Verification items for the finished model (mm, model axes). A direction names the side the tool comes from. Coordinates: 2 decimals unless noted, no trailing zeros. Write each loop counter-clockwise with the first axis right and the second up, starting at its lowest first coordinate (ties: lowest second). Pieces come first, ordered by that corner, then holes. Notation, with made-up numbers: (2.5, 14.25) -> (52.5, 14.25) arc R22 cw to (52.5, 44.25) -> close; hole circle Ø3 at (19, -6). An arc over 180 degrees is marked (long way). Answer in a Markdown table with one row per item.
```python
from build123d import *

# Parameters (mm, degrees)
BASE_DEPTH                           = 8.2
SIDES_DEPTH                          = 21
F_3_2_3_2_MOUNTING_HOLES_D           = 3.2
F_3_2_3_2_MOUNTING_HOLES_ON_FACE_2_D = 3.2
F_3_2_3_2_MOUNTING_HOLES_ON_FACE_3_D = 3.2
INSIDEFILLET_R                       = 3
OUTSIDEFILLET_R                      = 4
NUTSLOT_START                        = -4
NUTSLOT_DEPTH                        = 3


with BuildPart() as part:
    # Sketch4 → Base (new body)
    with BuildSketch(Plane.XY):
        Polygon((0, 20), (0, 0), (20, 0), (20, 6), (6, 20), align=None)
    extrude(amount=BASE_DEPTH)

    # Sketch4_4 → Sides (add)
    with BuildSketch(Plane.XY):
        Polygon((0, 0), (20, 0), (20, 4), (4, 4), (4, 20), (0, 20), align=None)
    extrude(amount=SIDES_DEPTH)

    # 3.2 _3.2_ Mounting Holes (through all)
    with Locations(Plane(origin=(14, 0, 15), x_dir=(0, 0, -1), z_dir=(0, -1, 0))):
        with Locations((0, 0)):
            Hole(F_3_2_3_2_MOUNTING_HOLES_D / 2)

    # 3.2 _3.2_ Mounting Holes on face 2 (through all)
    with Locations(Plane(origin=(0, 14, 15), x_dir=(0, 0, -1), z_dir=(-1, 0, 0))):
        with Locations((0, 0)):
            Hole(F_3_2_3_2_MOUNTING_HOLES_ON_FACE_2_D / 2)

    # 3.2 _3.2_ Mounting Holes on face 3 (through all)
    with Locations(Plane(origin=(9, 9, 0), x_dir=(-1, 0, 0), z_dir=(0, 0, -1))):
        with Locations((0, 0)):
            Hole(F_3_2_3_2_MOUNTING_HOLES_ON_FACE_3_D / 2)

    # InsideFillet
    insidefillet_edges = [part.edges().sort_by_distance(p)[0] for p in [
        (12, 4, 8.2),
        (4, 4, 14.6),
        (4, 12, 8.2),
    ]]
    fillet(insidefillet_edges, radius=INSIDEFILLET_R)

    # OutsideFillet
    outsidefillet_edges = [part.edges().sort_by_distance(p)[0] for p in [
        (6, 20, 4.185786438),
        (20, 6, 4.185786438),
        (20, 2, 21),
        (2, 20, 21),
    ]]
    fillet(outsidefillet_edges, radius=OUTSIDEFILLET_R)

    # Sketch7 → NutSlot (cut)
    with BuildSketch(Plane(origin=(0, 0, 0), x_dir=(-1, 0, 0), z_dir=(0, 0, -1)).offset(NUTSLOT_START)):
        Polygon((-8.228417185, 17.771582815), (-5.641242789, 8.116116524), (-8.116116524, 5.641242789), (-17.771582815, 8.228417185), align=None)
    extrude(amount=-NUTSLOT_DEPTH, mode=Mode.SUBTRACT)


solid = part.part
```
1. Tool access check on faces 4 (the flat face through (10.3, 10.4, 7)), 5 (the flat face through (13, 13, 3)), 6 (the flat face through (4, 13, 17)). Record the directions out of +Z, -Z, +X, -X, +Y, -Y that give a thin tool (end or side, any length) a straight path to the whole face; none if there is none.
Geometry says:
| item | result |
|---|---|
| face 4 | none |
| face 5 | +Z, -Z, +X, +Y |
| face 6 | +Z, +X, +Y |
2. Section check D-D, the plane y = 14. Record the boundary of the cut face in (x, z), plus the area to 3 significant figures.
Geometry says:
| item | result |
|---|---|
| outline | (0, 0) -> (12, 0) -> (12, 4) -> (7.22, 4) -> (7.22, 7) -> (12, 7) -> (12, 8.2) -> (7, 8.2) arc R3 cw to (4, 11.2) -> (4, 13.4) -> (0, 13.4) -> close; (0, 16.6) -> (4, 16.6) -> (4, 21) -> (0, 21) -> close |
| area | 124 mm^2 |
3. Depth check by flat-ended pin: P1, Ø8, axis at x = 12, z = 8, coming from the +Y side; P2, Ø9.5, axis at x = 15, y = 12, coming from the +Z side; P3, Ø5, axis at x = 11.5, z = 14.5, coming from the +Y side. Enter the tip coordinate at first touch or a pass-through.
Geometry says:
| item | result |
|---|---|
| P1 | y = 18 |
| P2 | z = 8.2 |
| P3 | y = 4 |
4. Thickness scan on line 1 (Y direction, x = 9, z = 7.7); line 2 (Z direction, x = 10.25, y = 11); line 3 (X direction, y = 2.4, z = 15). Record the ranges inside material, lowest first. Write a range as from..to.
Geometry says:
| item | result |
|---|---|
| line 1 | 0..7.4, 10.6..17 |
| line 2 | 0..4, 7..8.2 |
| line 3 | 0..12.4, 15.6..20 |
5. Section check B-B, the plane y = 9. Record the boundary of the cut face in (x, z), plus the area to 3 significant figures.
Geometry says:
| item | result |
|---|---|
| outline | (0, 0) -> (7.4, 0) -> (7.4, 4) -> (5.88, 4) -> (5.88, 7) -> (7.4, 7) -> (7.4, 8.2) -> (7, 8.2) arc R3 cw to (4, 11.2) -> (4, 21) -> (0, 21) -> close; (10.6, 0) -> (17, 0) -> (17, 4) -> (10.6, 4) -> close; (10.6, 7) -> (17, 7) -> (17, 8.2) -> (10.6, 8.2) -> close |
| area | 143 mm^2 |
6. Section check A-A, the plane z = 15. Record the boundary of the cut face in (x, y).
Geometry says:
| item | result |
|---|---|
| outline | (0, 0) -> (12.4, 0) -> (12.4, 4) -> (7, 4) arc R3 cw to (4, 7) -> (4, 12.4) -> (0, 12.4) -> close; (0, 15.6) -> (4, 15.6) -> (4, 20) -> (0, 20) -> close; (15.6, 0) -> (20, 0) -> (20, 4) -> (15.6, 4) -> close |
7. Mould release check, pull along X, two halves, no side actions. Record for faces 1 (the cylindrical face through (5.854, 19.704, 3.882)), 2 (the cylindrical face through (13.59, 4.9, 9.06)), 3 (the flat face through (10.3, 10.4, 4)): released by +X, released by -X, zero draft, split by the parting line, or undercut.
Geometry says:
| item | result |
|---|---|
| face 1 | released by +X |
| face 2 | zero draft |
| face 3 | undercut |
